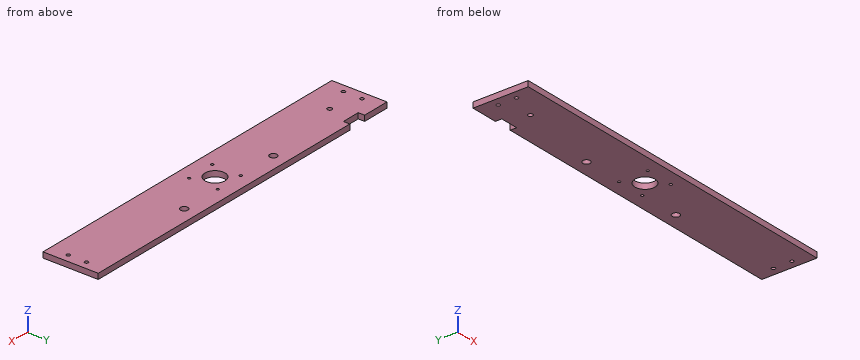
from build123d import *

# Parameters (mm, degrees)
SKETCH1_R           = 2
SKETCH1_R_2         = 2.5
SKETCH1_R_3         = 4
SKETCH1_R_4         = 11
BOSS_EXTRUDE1_DEPTH = 6
CUT_EXTRUDE1_REACH  = 8
SKETCH2_R           = 1.5


with BuildPart() as part:
    # Sketch1 → Boss-Extrude1 (new body)
    with BuildSketch(Plane.XY):
        Polygon((-194, 30), (-194, -30), (194, -30), (194, 30), (-144, 30), (-144, 23), (-164, 23), (-164, 30), align=None)
        with Locations((-185, -10)):
            Circle(SKETCH1_R, mode=Mode.SUBTRACT)
        with Locations((185, -10)):
            Circle(SKETCH1_R, mode=Mode.SUBTRACT)
        with Locations((-154, 0)):
            Circle(SKETCH1_R_2, mode=Mode.SUBTRACT)
        with Locations((-185, 10)):
            Circle(SKETCH1_R, mode=Mode.SUBTRACT)
        with Locations((-60, 15)):
            Circle(SKETCH1_R_3, mode=Mode.SUBTRACT)
        Circle(SKETCH1_R_4, mode=Mode.SUBTRACT)
        with Locations((60, 15)):
            Circle(SKETCH1_R_3, mode=Mode.SUBTRACT)
        with Locations((185, 10)):
            Circle(SKETCH1_R, mode=Mode.SUBTRACT)
    extrude(amount=BOSS_EXTRUDE1_DEPTH)

    # Sketch2 → Cut-Extrude1 (cut, up to next)
    with BuildSketch(Plane.XY.offset(6), mode=Mode.PRIVATE) as cut_extrude1_sk1:
        with Locations((15.495, 15.495)):
            Circle(SKETCH2_R)
    cut_extrude1_tool1 = extrude(cut_extrude1_sk1.sketch, amount=-CUT_EXTRUDE1_REACH, mode=Mode.PRIVATE) & part.part
    add(cut_extrude1_tool1.solids().sort_by_distance((15.495, 15.495, 6))[0], mode=Mode.SUBTRACT)
    # Sketch2 → Cut-Extrude1 (cut, up to next)
    with BuildSketch(Plane.XY.offset(6), mode=Mode.PRIVATE) as cut_extrude1_sk2:
        with Locations((-15.495, 15.495)):
            Circle(SKETCH2_R)
    cut_extrude1_tool2 = extrude(cut_extrude1_sk2.sketch, amount=-CUT_EXTRUDE1_REACH, mode=Mode.PRIVATE) & part.part
    add(cut_extrude1_tool2.solids().sort_by_distance((-15.495, 15.495, 6))[0], mode=Mode.SUBTRACT)
    # Sketch2 → Cut-Extrude1 (cut, up to next)
    with BuildSketch(Plane.XY.offset(6), mode=Mode.PRIVATE) as cut_extrude1_sk3:
        with Locations((15.495, -15.495)):
            Circle(SKETCH2_R)
    cut_extrude1_tool3 = extrude(cut_extrude1_sk3.sketch, amount=-CUT_EXTRUDE1_REACH, mode=Mode.PRIVATE) & part.part
    add(cut_extrude1_tool3.solids().sort_by_distance((15.495, -15.495, 6))[0], mode=Mode.SUBTRACT)
    # Sketch2 → Cut-Extrude1 (cut, up to next)
    with BuildSketch(Plane.XY.offset(6), mode=Mode.PRIVATE) as cut_extrude1_sk4:
        with Locations((-15.495, -15.495)):
            Circle(SKETCH2_R)
    cut_extrude1_tool4 = extrude(cut_extrude1_sk4.sketch, amount=-CUT_EXTRUDE1_REACH, mode=Mode.PRIVATE) & part.part
    add(cut_extrude1_tool4.solids().sort_by_distance((-15.495, -15.495, 6))[0], mode=Mode.SUBTRACT)


solid = part.part
Geometry check sheet. Reference: the model listing, model coordinates, mm. Give positions to 0.01 mm unless a question says otherwise; leave off trailing zeros. Order: outer loops, then holes, each group sorted by start corner. A loop starts at its lowest first (then second) coordinate and runs counter-clockwise, first axis right, second up.
1. Sectioned sample at B-B (z = 1.7). State how many separate pieces and enclosed holes the cut face has, then the cut area to 3 significant figures.
Completed:
separate pieces: 1
enclosed holes: 12
area: 22,600 mm2
2. Depth check by flat-ended pin: pin 1 (5 mm diameter, centred on x = -93.5, y = 11, fed in from -Z); pin 2 (3 mm diameter, centred on x = 185, y = 10, fed in from +Z); pin 3 (3 mm diameter, centred on x = -157, z = 2.5, fed in from +Y). Enter the tip coordinate at first touch or a pass-through.
Completed:
pin 1: stops at z = 0
pin 2: passes through
pin 3: stops at y = 23
3. Sectioned sample at A-A (x = 0). Record the boundary of the cut face in (y, z), then the cut area to 3 significant figures.
Completed:
outline: (-30, 0) - (-11, 0) - (-11, 6) - (-30, 6) - close; (11, 0) - (30, 0) - (30, 6) - (11, 6) - close
area: 228 mm2
4. Sectioned sample at C-C (x = -60). Record the boundary of the cut face in (y, z).
Completed:
outline: (-30, 0) - (11, 0) - (11, 6) - (-30, 6) - close; (19, 0) - (30, 0) - (30, 6) - (19, 6) - close
5. Scan lines: line 1 (Y direction, x = -185, z = 3.9); line 2 (X direction, y = -15.5, z = 4.5) (3 decimals); line 3 (Y direction, x = -60, z = 2.5). Record each from-to range of solid material in increasing order.
Completed:
line 1: y = -30 to -12, -8 to 8, 12 to 30
line 2: x = -194 to -16.995, -13.995 to 13.995, 16.995 to 194
line 3: y = -30 to 11, 19 to 30
